Autodesk Inventor part; units mm, degrees
ref_plane "YZ Plane" through (0, 0, 0) normal (1, 0, 0) x (0, 1, 0)
ref_plane "XZ Plane" through (0, 0, 0) normal (0, 1, 0) x (-1, 0, 0)
ref_plane "XY Plane" through (0, 0, 0) normal (0, 0, 1) x (1, 0, 0)
sketch "Skizze1" plane through (0, 0, 0) normal (0, 0, 1) x (1, 0, 0)
  line L0 (0, 0) -> (16.6, 0)
  line L1 (16.6, 0) -> (16.6, 11.45)
  line L2 (16.6, 11.45) -> (0, 11.45)
  line L3 (0, 11.45) -> (0, 0)
  line L4 (16.6, 0) -> (20.7, 0)
  line L5 (20.7, 0) -> (20.7, 11.15)
  line L6 (20.7, 11.15) -> (16.6, 11.15)
  line L7 (16.6, 11.15) -> (16.6, 0)
  line L8 (20.7, 0) -> (23.1, 0)
  line L9 (23.1, 0) -> (23.1, 11.45)
  line L10 (23.1, 11.45) -> (20.7, 11.45)
  line L11 (20.7, 11.45) -> (20.7, 0)
  line L12 (23.1, 0) -> (32.4, 0)
  line L13 (32.4, 0) -> (32.4, 13.6)
  line L14 (32.4, 13.6) -> (23.1, 13.6)
  line L15 (23.1, 13.6) -> (23.1, 0)
  dimension "d1" = 11.45
  dimension "d2" = 4.1
  dimension "d3" = 11.15
  dimension "d4" = 2.4
  dimension "d5" = 9.3
  dimension "d6" = 13.6
  dimension "d8" = 32.4
revolve "Umdrehung1" add sketch "Skizze1" angle 360 about axis through (0, 0, 0) along (1, 0, 0)
properties part number "00_Eyepiece_WF20x 23,2mm"
Read the model definition and answer for the solid it produces. Units are mm, in the model's axes. A direction names the side the tool comes from. Give positions to 0.01 mm unless a question says otherwise; leave off trailing zeros. Write each loop counter-clockwise with the first axis right and the second up, starting at its lowest first coordinate (ties: lowest second). Pieces come first, ordered by that corner, then holes. Notation, with made-up numbers: M 28,-5 L 33,-5 A25 ccw 33,28 Z; hole C 53.25,-31.75 d4. An arc over 180 degrees is marked long. Put each result on its own line as item: value. Start each with the question number.
1. Consider line 1 along X through (y, z) = (2, -11); line 2 along X through (y, z) = (11.25, -4.5); line 3 along Y through (x, z) = (2.5, -10.25). Determine where each line is inside the solid, lowest interval first.
2. The part is cut by section D-D, the plane x = 3. Give the vertices of the cut face in (y, z), and give its area (3 significant figures).
3. The part is cut by section C-C, the plane x = 25. Give the vertices of the cut face in (y, z).
4. The part is cut by section A-A, the plane y = 0. Give the vertices of the cut face in (x, z), and give its area (3 significant figures).
5. Each of these flat-tipped pins is pushed along its axis until it touches: pin 1 Ø1 at (y, z) = (-6, 6) entering from -X; pin 2 Ø5 at (x, y) = (13, 0.5) entering from -Z; pin 3 Ø1.5 at (x, y) = (3.5, 4) entering from +Z; pin 4 Ø6 at (x, z) = (18.5, -2.5) entering from -Y. Where does it stop, or does it pass through?
6. For a pull along X with two mould halves and no side action, classify faces 1 (the flat face through (23.1, -6, -10)), 2 (the flat face through (32.4, 0, 0)), 3 (the cylindrical face through (21.88, -2.48, 11.18)), 4 (the cylindrical face through (18.621, 10.635, -3.349)) as released by +X, released by -X, zero draft, split by the parting line, or undercut.
7. Which of the six approach directions +Z, -Z, +X, -X, +Y, -Y give full straight-line access (tool end or side, diameter ignored) to faces 5 (the cylindrical face through (8.18, -2.48, 11.18)), 6 (the flat face through (0, 0, 0))?
Final values:
1. line 1: x = 0 to 16.6, 20.7 to 32.4
1. line 2: x = 23.1 to 32.4
1. line 3: y = -5.1 to 5.1
2. outline: C 0,0 d22.9
2. area: 412 mm²
3. outline: C 0,0 d27.2
4. outline: M 0,-11.45 L 16.6,-11.45 L 16.6,-11.15 L 20.7,-11.15 L 20.7,-11.45 L 23.1,-11.45 L 23.1,-13.6 L 32.4,-13.6 L 32.4,13.6 L 23.1,13.6 L 23.1,11.45 L 20.7,11.45 L 20.7,11.15 L 16.6,11.15 L 16.6,11.45 L 0,11.45 Z
4. area: 779 mm²
5. pin 1: stops at x = 0
5. pin 2: stops at z = -11.45
5. pin 3: stops at z = 10.98
5. pin 4: stops at y = -11.45
6. face 1: released by -X
6. face 2: released by +X
6. face 3: zero draft
6. face 4: undercut
7. face 5: -X
7. face 6: +Z, -Z, -X, +Y, -Y
